```python
from build123d import *

# Parameters (mm, degrees)
F0_W     = 50
F0_H     = 50
F0_W_2   = 40
F0_H_2   = 40
F1_DEPTH = 30
F2_W     = 50
F2_H     = 50
F3_DEPTH = 25
F4_SIZE  = 24.99999
F5_W     = 10
F5_H     = 16
F6_DEPTH = 5
F5_W_2   = 7
F5_H_2   = 7
F7_DEPTH = 50.001
F5_R     = 4.5
F8_DEPTH = 50.001


# Not quite as in the source:
# - a fillet or chamfer is up to 0.001 mm smaller than in the source, because OpenCascade refuses the exact size


with BuildPart() as f1:
    # F0 (on Top) → F1 (new body)
    with BuildSketch(Plane.XY):
        with Locations((25, 25)):
            Rectangle(F0_W, F0_H)
        with Locations((25, 25)):
            Rectangle(F0_W_2, F0_H_2, mode=Mode.SUBTRACT)
    extrude(amount=F1_DEPTH)

    # F2 (on face) → F3 (join)
    with BuildSketch(Plane.XY.offset(30)):
        with Locations((25, 25)):
            Rectangle(F2_W, F2_H)
    extrude(amount=F3_DEPTH)

    # F4 (size 25 in the source; OpenCascade refuses exactly that, so slightly less here)
    f4_edges = [f1.edges().sort_by_distance(p)[0] for p in [
        (0, 25, 55),
        (50, 25, 55),
    ]]
    chamfer(f4_edges, length=F4_SIZE)

    # F5 (on face) → F6 (cut)
    with BuildSketch(Plane.XZ):
        with Locations((23.930438906, 8)):
            Rectangle(F5_W, F5_H)
    extrude(amount=-F6_DEPTH, mode=Mode.SUBTRACT)

    # F5 (on face) → F7 (cut, through all)
    with BuildSketch(Plane.XZ):
        with Locations((10.5, 26.0614674687)):
            Rectangle(F5_W_2, F5_H_2)
        with Locations((39.5, 26.5)):
            Rectangle(F5_W_2, F5_H_2)
    extrude(amount=-F7_DEPTH, mode=Mode.SUBTRACT)

    # F5 (on face) → F8 (cut, through all)
    with BuildSketch(Plane.XZ):
        with Locations((25, 41.7942066526)):
            Circle(F5_R)
    extrude(amount=-F8_DEPTH, mode=Mode.SUBTRACT)


solid = f1.part
```
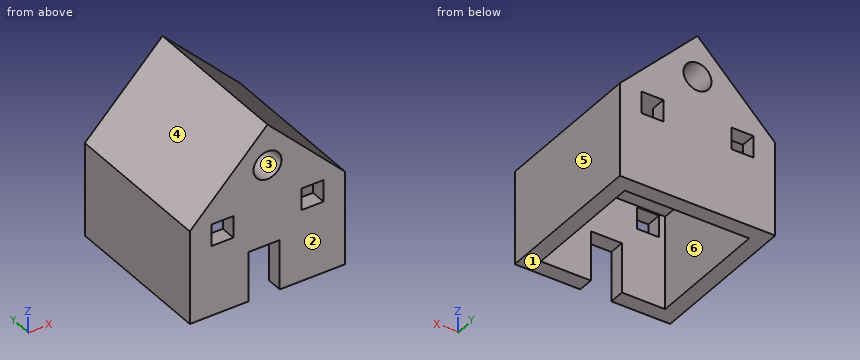
Check sheet for the modelled part. Datum: model origin and axes. Units: mm. Face numbers are marked on the shaded views. A direction names the side the tool comes from. Round coordinates to 2 decimals unless told otherwise and drop trailing zeros. Order: outer loops, then holes, each group sorted by start corner. A loop starts at its lowest first (then second) coordinate and runs counter-clockwise, first axis right, second up. Notation, with made-up numbers: (9, 30) - (20, 30) arc R14 ccw to (20, 39) - close; hole circle Ø1 at (2, -20). An arc over 180 degrees is marked (long way). Write item = value, one per line.
Q1. Draft check along Z on the marked faces 1, 2, 3 and 4. Enter one of: pulls with the +Z half, pulls with the -Z half, needs draft (parallel to the pull), parting line crosses it, or undercut.
Computed:
face_1 = pulls with the -Z half
face_2 = needs draft
face_3 = undercut
face_4 = pulls with the +Z half
Q2. Tool access check on the marked faces 5 and 6. Record the directions out of +Z, -Z, +X, -X, +Y, -Y that give a thin tool (end or side, any length) a straight path to the whole face; none if there is none.
Computed:
face_5 = +Z, -Z, +X, +Y, -Y
face_6 = -Z
Q3. Section check C-C (x = 18). Record the boundary of the cut face in (y, z), and give its area (3 significant figures).
Computed:
outline = (0, 0) - (5, 0) - (5, 30) - (45, 30) - (45, 0) - (50, 0) - (50, 48) - (0, 48) - close
area = 1,200 mm^2
Q4. Section check A-A (z = 20.5). Record the boundary of the cut face in (x, y), and give its area (3 significant figures).
Computed:
outline = (0, 0) - (50, 0) - (50, 50) - (0, 50) - close; hole (5, 5) - (45, 5) - (45, 45) - (5, 45) - close
area = 900 mm^2
Q5. Section check B-B (z = 12.5). Record the boundary of the cut face in (x, y), and give its area (3 significant figures).
Computed:
outline = (0, 0) - (18.93, 0) - (18.93, 5) - (5, 5) - (5, 45) - (45, 45) - (45, 5) - (28.93, 5) - (28.93, 0) - (50, 0) - (50, 50) - (0, 50) - close
area = 850 mm^2
Q6. Thickness scan on line 1 along Y through (x, z) = (21.5, 21); line 2 along Z through (x, y) = (25, 27). Record the ranges inside material, lowest first.
Computed:
line_1 = 0 to 5, 45 to 50
line_2 = 30 to 37.29, 46.29 to 55
Q7. Go/stop test with flat-tipped pins: pin 1 (8 mm diameter, centred on x = 8.5, y = 12.5, fed in from +Z); pin 2 (1.5 mm diameter, centred on x = 40.5, y = 48, fed in from +Z); pin 3 (4 mm diameter, centred on x = 10, y = 47, fed in from +Z). Record where each tip stops, or that it passes through.
Computed:
pin_1 = 42.5
pin_2 = 40.25
pin_3 = 42
